Autodesk Inventor part; units mm, degrees
ref_plane "YZ Plane" through (0, 0, 0) normal (1, 0, 0) x (0, 1, 0)
ref_plane "XZ Plane" through (0, 0, 0) normal (0, 1, 0) x (-1, 0, 0)
ref_plane "XY Plane" through (0, 0, 0) normal (0, 0, 1) x (1, 0, 0)
sketch "Sketch1" plane through (0, 0, 0) normal (0, 1, 0) x (-1, 0, 0)
  line L0 (0, 0) -> (17.9, 0)
  line L1 (17.9, 0) -> (17.9, -64.8)
  line L2 (17.9, -64.8) -> (0, -64.8)
  line L3 (0, -64.8) -> (0, 0)
  line L4 (17.9, -14.6) -> (31.9, -14.6)
  line L5 (31.9, -14.6) -> (31.9, -17.6)
  line L6 (31.9, -17.6) -> (17.9, -17.6)
  line L7 (17.9, -17.6) -> (17.9, -14.6)
  line L8 (17.9, -22.4) -> (31.9, -22.4)
  line L9 (31.9, -22.4) -> (31.9, -42.4)
  line L10 (31.9, -42.4) -> (17.9, -42.4)
  line L11 (17.9, -42.4) -> (17.9, -22.4)
  line L12 (17.9, -47.2) -> (31.9, -47.2)
  line L13 (31.9, -47.2) -> (31.9, -50.2)
  line L14 (31.9, -50.2) -> (17.9, -50.2)
  line L15 (17.9, -50.2) -> (17.9, -47.2)
  line L16 (47.989, -20) -> (-6.1915, -20) construction
  line L17 (47.989, -44.8) -> (-4.845, -44.8) construction
  line L18 (0, -50.2) -> (-1.5, -50.2)
  line L19 (-1.5, -50.2) -> (-1.5, -14.6)
  line L20 (-1.5, -14.6) -> (0, -14.6)
  line L21 (0, -14.6) -> (0, -50.2)
  point P0 (17.9, -42.4)
  point P1 (0, -14.6)
  dimension "d0" = 17.9
  dimension "d2" = 3
  dimension "d4" = 20
  dimension "d5" = 24.8
  dimension "d6" = 2.4
  dimension "d7" = 2.4
  dimension "d8" = 2.4
  dimension "d9" = 2.4
  dimension "d10" = 3
  dimension "d11" = 14
  dimension "d14" = 20
  dimension "d24" = 1.5
extrude "Extrusion1" add sketch "Sketch1" along normal blind 17.9
fillet "Fillet1" radius 2 16 edges at (-17.9, 8.95, -64.8) (-8.95, 0, -64.8) (0, 8.95, -64.8) (-8.95, 17.9, -64.8) (-8.95, 17.9, 0) (-17.9, 8.95, 0) (-8.95, 0, 0) (0, 8.95, 0) (0, 17.9, -7.3) (0, 17.9, -57.5) (0, 0, -7.3) (0, 0, -57.5) (-17.9, 17.9, -57.5) (-17.9, 0, -57.5) (-17.9, 17.9, -7.3) (-17.9, 0, -7.3)
sketch "Sketch2" plane through (-31.9, 0, -14.6) normal (0, 0, 1) x (1, 0, 0)
  circle A0 centre (4, 13.9) radius 1.6
  circle A1 centre (4, 4) radius 1.6
  line L0 (14, 15.9) -> (14, 2)
  line L1 (0, 0) -> (16, 0)
  line L2 (0, 17.9) -> (16, 17.9)
  point P0 (31.9, 0)
  point P1 (14, 17.8)
  point P2 (14, 0)
  point P3 (12, 0)
  point P4 (12, 17.8)
  point P5 (12.5359, 0)
  point P6 (12.5359, 17.8)
  point P7 (16, 17.9)
  dimension "d16" = 3.2
  dimension "d17" = 3.2
  dimension "d18" = 10
  dimension "d19" = 10
  dimension "d20" = 4
  dimension "d21" = 4
extrude "Extrusion2" cut sketch "Sketch2" against normal blind 100
ref_plane "Work Plane1" through (0, 8.95, 0) normal (0, 1, 0) x (1, 0, 0)
equation "\"d7\" = d6"
equation "\"d8\" = d6"
equation "\"d9\" = d6"
equation "\"d19\" = d18"
properties part number "Square_tube_connector"
Verification items for the finished model (mm, model axes). A direction names the side the tool comes from. Give positions to 0.01 mm unless a question says otherwise; leave off trailing zeros. Order: outer loops, then holes, each group sorted by start corner. A loop starts at its lowest first (then second) coordinate and runs counter-clockwise, first axis right, second up. Notation, with made-up numbers: (14, 42) - (46, 42) arc R24 cw to (46, 54) - close; hole circle Ø10 at (37.5, -16). An arc over 180 degrees is marked (long way). Answer as CSV lines item,"result". Start each with the question number.
Item 1: Section check B-B, the plane z = -30. Record the boundary of the cut face in (x, y).
Item 2: Material ranges on L1, parallel to Z at x = -23, y = 2; L2, parallel to Y at x = -27.9, z = -33.75; L3, parallel to Y at x = -27, z = -49, recorded low to high.
Item 3: Section check D-D, the plane z = -9. Record the boundary of the cut face in (x, y).
Item 4: Mould release check, pull along X, two halves, no side actions. Record for faces 1 (the face through (-17.9, 9, -20)), 2 (the face through (-29.5, 4.07, -16.08)), 3 (the face through (0, 9, -8)): released by +X, released by -X, zero draft, split by the parting line, or undercut.
Item 5: Section check A-A, the plane x = -25. Record the boundary of the cut face in (y, z), plus the area to 3 significant figures.
Item 6: Access from +Z, -Z, +X, -X, +Y, -Y to the whole of each face (thin tool, end or side, straight path). Record for faces 4 (the face through (0, 9, -57)), 5 (the face through (-17.9, 9, -8)), 6 (the face through (-29.5, 13.97, -48.68)), 7 (the face through (-0.57, 17.3, -8.21)), 8 (the face through (-17.9, 9, -45)).
Item 7: Gauge pin test, flat ends, axial feed: pin 1 (5 mm diameter, centred on x = -23, y = 10.5, fed in from +Z); pin 2 (4 mm diameter, centred on y = 7.5, z = -55.5, fed in from -X); pin 3 (5 mm diameter, centred on x = -20, y = 6, fed in from -Z). Record the tip position at first contact, or that the pin passes through.
Item 8: Section check C-C, the plane y = 7. Record the boundary of the cut face in (x, z), plus the area to 3 significant figures.
Filled in:
1,outline,"(-31.9, 0) - (1.5, 0) - (1.5, 17.9) - (-31.9, 17.9) - close; hole circle Ø3.2 at (-27.9, 4); hole circle Ø3.2 at (-27.9, 13.9)"
2,L1,"-50.2 to -47.2, -42.4 to -22.4, -17.6 to -14.6"
2,L2,"0 to 2.4, 5.6 to 12.3, 15.5 to 17.9"
2,L3,"0 to 2.68, 5.32 to 12.58, 15.22 to 17.9"
3,outline,"(-17.9, 2) arc R2 ccw to (-15.9, 0) - (-2, 0) arc R2 ccw to (0, 2) - (0, 15.9) arc R2 ccw to (-2, 17.9) - (-15.9, 17.9) arc R2 ccw to (-17.9, 15.9) - close"
4,face 1,"released by -X"
4,face 2,"undercut"
4,face 3,"released by +X"
5,outline,"(0, -50.2) - (17.9, -50.2) - (17.9, -47.2) - (0, -47.2) - close; (0, -42.4) - (17.9, -42.4) - (17.9, -22.4) - (0, -22.4) - close; (0, -17.6) - (17.9, -17.6) - (17.9, -14.6) - (0, -14.6) - close"
5,area,"465 mm^2"
6,face 4,"-Z, +X, +Y, -Y"
6,face 5,"+Z, -X, +Y, -Y"
6,face 6,"+Z, -Z"
6,face 7,"+Z, +X, +Y"
6,face 8,"-X, +Y, -Y"
7,pin 1,"z = -14.6"
7,pin 2,"x = -17.9"
7,pin 3,"z = -64"
8,outline,"(-31.9, -50.2) - (-17.9, -50.2) - (-17.9, -62.8) arc R2 ccw to (-15.9, -64.8) - (-2, -64.8) arc R2 ccw to (0, -62.8) - (0, -50.2) - (1.5, -50.2) - (1.5, -14.6) - (0, -14.6) - (0, -2) arc R2 ccw to (-2, 0) - (-15.9, 0) arc R2 ccw to (-17.9, -2) - (-17.9, -14.6) - (-31.9, -14.6) - (-31.9, -17.6) - (-17.9, -17.6) - (-17.9, -22.4) - (-31.9, -22.4) - (-31.9, -42.4) - (-17.9, -42.4) - (-17.9, -47.2) - (-31.9, -47.2) - close"
8,area,"1,570 mm^2"
